The listing builds one solid part. Answer for the finished solid, in the listing's coordinates (mm). A direction names the side the tool comes from. Give positions to 0.01 mm unless a question says otherwise; leave off trailing zeros. Write each loop counter-clockwise with the first axis right and the second up, starting at its lowest first coordinate (ties: lowest second). Pieces come first, ordered by that corner, then holes. Notation, with made-up numbers: (49, 84) -> (107, 84) arc R14 cw to (107, 98) -> close; hole circle Ø10 at (21.25, -15.75). An arc over 180 degrees is marked (long way). One line per question, with ' | ' between items.
from build123d import *

# Parameters (mm, degrees)
SKETCH_2_W            = 28.5
SKETCH_2_H            = 52
SKETCH_2_R            = 1.5
EXTRUDE_1_DEPTH       = 1.5
EXTRUDE_START         = 4.65
EXTRUDE_2_DEPTH       = 19.2
EXTRUDE_2_2_OUTLINE_W = 1
EXTRUDE_2_2_OUTLINE_H = 38.620640838
EXTRUDE_2_2_DEPTH     = 2.24290402
EXTRUDE_START_2       = 26.25709598
EXTRUDE_2_3_OUTLINE_W = 1
EXTRUDE_2_3_OUTLINE_H = 38.620640838
EXTRUDE_2_3_DEPTH     = 2.24290402
EXTRUDE_START_3       = 9.75
EXTRUDE_2_4_OUTLINE_W = 3
EXTRUDE_2_4_OUTLINE_H = 1.7
EXTRUDE_2_4_DEPTH     = 9
EXTRUDE_START_4       = 3.7
EXTRUDE_2_5_OUTLINE_W = 3
EXTRUDE_2_5_OUTLINE_H = 5.3
EXTRUDE_2_5_DEPTH     = 20.8


# Read off the part's stored shape, not the designer's step: Бобышка-Вытянуть2
with BuildPart() as part:
    # Эскиз2 → Бобышка-Вытянуть1 (new body)
    with BuildSketch(Plane(origin=(0, 0, 0), x_dir=(1, 0, 0), z_dir=(0, 1, 0))):
        with Locations((14.25, -26)):
            Rectangle(SKETCH_2_W, SKETCH_2_H)
        with Locations(Location((2.2, -2, 0), (0, 0, 270))):
            Circle(SKETCH_2_R, mode=Mode.SUBTRACT)
        with Locations(Location((26, -2, 0), (0, 0, 270))):
            Circle(SKETCH_2_R, mode=Mode.SUBTRACT)
        with Locations(Location((2.2, -50, 0), (0, 0, 90))):
            Circle(SKETCH_2_R, mode=Mode.SUBTRACT)
        with Locations(Location((26, -49.8, 0), (0, 0, 270))):
            Circle(SKETCH_2_R, mode=Mode.SUBTRACT)
    extrude(amount=EXTRUDE_1_DEPTH)

    # Бобышка-Вытянуть2 outline → Бобышка-Вытянуть2 (add)
    with BuildSketch(Plane.YZ.offset(EXTRUDE_START)):
        Polygon((4.5, 52), (1.5, 52), (1.5, 7), (3.5, 7), (3.5, 46.7), (4.5, 46.7), align=None)
    extrude(amount=EXTRUDE_2_DEPTH)

    # Extrude 2 2 outline → Extrude 2 2 (add)
    with BuildSketch(Plane.YZ):
        with Locations((2, 24.067488006)):
            Rectangle(EXTRUDE_2_2_OUTLINE_W, EXTRUDE_2_2_OUTLINE_H)
    extrude(amount=EXTRUDE_2_2_DEPTH)

    # Extrude 2 3 outline → Extrude 2 3 (add)
    with BuildSketch(Plane.YZ.offset(EXTRUDE_START_2)):
        with Locations((2, 24.067488006)):
            Rectangle(EXTRUDE_2_3_OUTLINE_W, EXTRUDE_2_3_OUTLINE_H)
    extrude(amount=EXTRUDE_2_3_DEPTH)

    # Extrude 2 4 outline → Extrude 2 4 (add)
    with BuildSketch(Plane.YZ.offset(EXTRUDE_START_3)):
        with Locations((3, 52.85)):
            Rectangle(EXTRUDE_2_4_OUTLINE_W, EXTRUDE_2_4_OUTLINE_H)
    extrude(amount=EXTRUDE_2_4_DEPTH)

    # Extrude 2 5 outline → Extrude 2 5 (add)
    with BuildSketch(Plane.YZ.offset(EXTRUDE_START_4)):
        with Locations((3, 49.35)):
            Rectangle(EXTRUDE_2_5_OUTLINE_W, EXTRUDE_2_5_OUTLINE_H)
    extrude(amount=EXTRUDE_2_5_DEPTH)


solid = part.part
Item 1: Find section C-C (x = 11). Write down the section's boundary in (y, z).
Answers below:
outline: (0, 0) -> (1.5, 0) -> (1.5, 7) -> (3.5, 7) -> (3.5, 46.7) -> (4.5, 46.7) -> (4.5, 53.7) -> (1.5, 53.7) -> (1.5, 52) -> (0, 52) -> close
Item 2: Determine the mould class of faces 4 (the face through (14, 1, 52)), 5 (the face through (26.257, 2, 24)), 6 (the face through (14, 2, 7)), 7 (the face through (9.75, 3, 53)) for opening direction X: pulls with the +X half, pulls with the -X half, needs draft (parallel to the pull), parting line crosses it, or undercut.
Answers below:
face 4: needs draft | face 5: undercut | face 6: undercut | face 7: pulls with the -X half
Item 3: Consider line 1 (X direction, y = 1.15, z = 2); line 2 (Y direction, x = 2.5, z = 30.5); line 3 (Z direction, x = 6.75, y = 3.7). Determine where each line is inside the solid, lowest interval first. Write a range as [from, to].
Answers below:
line 1: [0, 0.7], [3.7, 24.5], [27.5, 28.5] | line 2: [0, 1.5] | line 3: [46.7, 52]
Item 4: Find section A-A (z = 2). Write down the section's boundary in (x, y), then the cut area to 4 significant figures.
Answers below:
outline: (0, 0) -> (0.7, 0) -> (0.7, 1.5) -> (0, 1.5) -> close; (3.7, 0) -> (24.5, 0) -> (24.5, 1.5) -> (3.7, 1.5) -> close; (27.5, 0) -> (28.5, 0) -> (28.5, 1.5) -> (27.5, 1.5) -> close | area: 33.75 mm²
Item 5: Find section D-D (z = 45). Write down the section's boundary in (x, y), then the cut area to 4 significant figures.
Answers below:
outline: (0, 0) -> (28.5, 0) -> (28.5, 1.5) -> (23.85, 1.5) -> (23.85, 3.5) -> (4.65, 3.5) -> (4.65, 1.5) -> (0, 1.5) -> close | area: 81.15 mm²
Item 6: Flat-ended cylindrical pins translate along their axes: pin 1 (1.8 mm diameter, centred on x = 26, z = 49.8, fed in from +Y); pin 2 (1 mm diameter, centred on x = 24, z = 42, fed in from +Y); pin 3 (2 mm diameter, centred on x = 25, y = 0.5, fed in from +Z); pin 4 (0.8 mm diameter, centred on x = 27.5, y = 2, fed in from -Z). Find the tip coordinate at first contact, or state that the pin passes through.
Answers below:
pin 1: through | pin 2: y = 3.5 | pin 3: z = 52 | pin 4: z = 4.76
Item 7: A tool of negligible diameter and unlimited length cuts with its end or side. For faces 1 (the face through (24.5, 3, 49)), 2 (the face through (4.65, 2, 27)), 3 (the face through (3.7, 3, 49)), from which of +Z, -Z, +X, -X, +Y, -Y can it reach the whole face along a straight path? Write none if from no direction.
Answers below:
face 1: +Z, -Z, +X, +Y | face 2: -Z, +Y | face 3: +Z, -Z, -X, +Y
Item 8: Find section B-B (y = 0.8). Write down the section's boundary in (x, z).
Answers below:
outline: (0, 0) -> (28.5, 0) -> (28.5, 52) -> (0, 52) -> close; hole circle Ø3 at (2.2, 2); hole circle Ø3 at (2.2, 50); hole circle Ø3 at (26, 2); hole circle Ø3 at (26, 49.8)
